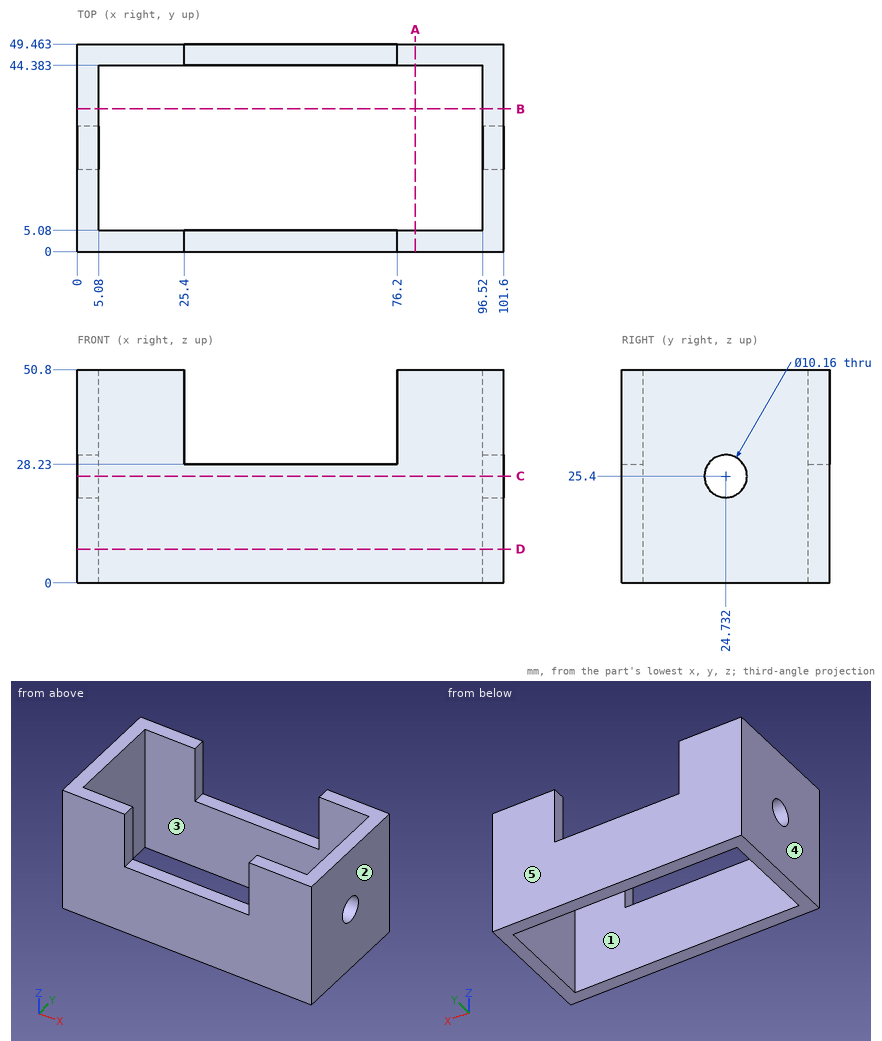
Source: three-view drawing plus pictorial views. Frame: mm from the lowest corner of the part. A direction names the side the tool comes from. Round coordinates to 2 decimals unless told otherwise and drop trailing zeros. Order: outer loops, then holes, each group sorted by start corner. A loop starts at its lowest first (then second) coordinate and runs counter-clockwise, first axis right, second up. Notation, with made-up numbers: (24, 26.25) - (65, 26.25) arc R14 cw to (65, 30.25) - close; hole circle Ø4 at (-37.75, -7). An arc over 180 degrees is marked (long way). Write each question's results on one line, items separated by ' | '.
Item 1: Mould query, pull axis Y, two halves, no side actions, for the marked faces 3, 4 and 5. Classes: pulls with the +Y half, pulls with the -Y half, needs draft (parallel to the pull), parting line crosses it, or undercut.
Completed:
face 3: undercut | face 4: needs draft | face 5: pulls with the +Y half
Item 2: Material intervals for line 1 along X through (y, z) = (45, 48); line 2 along X through (y, z) = (41, 35.5); line 3 along Y through (x, z) = (3, 25) (1 decimal), sorted ascending. Write a range as [from, to].
Completed:
line 1: [0, 25.4], [76.2, 101.6] | line 2: [0, 5.08], [96.52, 101.6] | line 3: [0, 19.7], [29.8, 49.5]
Item 3: Section D-D, the plane z = 8. Return the cut outline in (x, y), and give its area (3 significant figures).
Completed:
outline: (0, 0) - (101.6, 0) - (101.6, 49.46) - (0, 49.46) - close; hole (5.08, 5.08) - (96.52, 5.08) - (96.52, 44.38) - (5.08, 44.38) - close | area: 1,430 mm^2
Item 4: First-contact query: pin 1 Ø4 at (x, y) = (51, 3) entering from +Z. Flat tip, straight axial feed; report the tip coordinate or a pass-through.
Completed:
pin 1: z = 28.23
Item 5: Section C-C, the plane z = 25.4. Return the cut outline in (x, y), and give its area (3 significant figures).
Completed:
outline: (0, 0) - (101.6, 0) - (101.6, 19.65) - (96.52, 19.65) - (96.52, 5.08) - (5.08, 5.08) - (5.08, 19.65) - (0, 19.65) - close; (0, 29.81) - (5.08, 29.81) - (5.08, 44.38) - (96.52, 44.38) - (96.52, 29.81) - (101.6, 29.81) - (101.6, 49.46) - (0, 49.46) - close | area: 1,330 mm^2
Item 6: Reachability of the marked faces 1 and 2 from +Z, -Z, +X, -X, +Y, -Y: full face, straight path, thin tool, end or side. Return the list, or none.
Completed:
face 1: +Z, -Z | face 2: +Z, -Z, +X, +Y, -Y
Item 7: Section B-B, the plane y = 34. Return the cut outline in (x, z).
Completed:
outline: (0, 0) - (5.08, 0) - (5.08, 50.8) - (0, 50.8) - close; (96.52, 0) - (101.6, 0) - (101.6, 50.8) - (96.52, 50.8) - close
Item 8: Section A-A, the plane x = 80.5. Return the cut outline in (y, z), and give its area (3 significant figures).
Completed:
outline: (0, 0) - (5.08, 0) - (5.08, 50.8) - (0, 50.8) - close; (44.38, 0) - (49.46, 0) - (49.46, 50.8) - (44.38, 50.8) - close | area: 516 mm^2
